For this review, take the finished solid that the model builds, in its own axes (mm). A direction names the side the tool comes from. Round coordinates to 2 decimals unless told otherwise and drop trailing zeros. Order: outer loops, then holes, each group sorted by start corner. A loop starts at its lowest first (then second) coordinate and runs counter-clockwise, first axis right, second up. Notation, with made-up numbers: (19.25, 82) -> (53.25, 82) arc R22 cw to (53.25, 113) -> close; hole circle Ø3 at (71, 87). An arc over 180 degrees is marked (long way). Use a Markdown table: item, result. Add a question column.
1) Machinability: for faces 5 (the face through (-34.3, -493, -43)), 6 (the face through (0, -493, -55)), 7 (the face through (3, -1000, -54)), which of the approach directions +Z, -Z, +X, -X, +Y, -Y give a long, thin tool a straight path to every point of the face, cutting with its end or side? Answer none if there is none.
2) Wall thickness on line 1 along X through (y, z) = (-635, -70); line 2 along X through (y, z) = (-332.5, -45); line 3 along X through (y, z) = (-213, -13.5): over which ranges is each line inside the solid? List them lowest first. Write a range as [from, to].
3) Clearance check with flat-ended pins moving along their axes: P1, Ø2.5, axis at x = -33, y = -698.5, coming from the -Z side; P2, Ø1.6, axis at x = -35, y = -397, coming from the +Z side; P3, Ø2, axis at y = -471.5, z = -89.5, coming from the +X side. State where each tip first meets the part, or that it passes through.
4) Draft analysis for pull direction Z (two halves, no side actions). For faces 1 (the face through (-27.1, -493, -80)), 2 (the face through (-7, -493, -28)), 3 (the face through (-17, -493, -92)), 4 (the face through (21, -493, -53)), state which applies: pulls with the +Z half, pulls with the -Z half, needs draft (parallel to the pull), parting line crosses it, or undercut.
5) Consider section A-A (z = -44). State the section outline as (x, y) points, plus the area to 3 significant figures.
```python
from build123d import *

# Parameters (mm, degrees)
F1_DEPTH = 1000
F2_R     = 0.5
F5_DEPTH = 1000


with BuildPart() as f1:
    # F0 (on Front) → F1 (new body)
    with BuildSketch(Plane.XZ):
        Polygon((0, -5), (0, -3), (-7, -3), (-7, -53), (-34.3, -53), (-34.3, -33), (-36.3, -33), (-36.3, -61.5), (-34.3, -61.5), (-34.3, -55), (-29.1, -55), (-29.1, -75), (-34.3, -75), (-34.3, -68.5), (-36.3, -68.5), (-36.3, -77), (-29.1, -77), (-29.1, -92), (-5, -92), (-5, -88), (-7, -88), (-7, -90), (-27.1, -90), (-27.1, -69.9), (-25.1, -69.9), (-25.1, -67.9), (-27.1, -67.9), (-27.1, -55), (0, -55), (0, -53), (-5, -53), (-5, -5), align=None)
    extrude(amount=F1_DEPTH)

    # F2
    f2_edges = [f1.edges().sort_by_distance(p)[0] for p in [
        (-36.3, -500, -33),
        (-36.3, -500, -68.5),
        (-5, -500, -92),
        (-5, -500, -88),
        (-7, -500, -3),
        (-34.3, -500, -33),
        (-5, -500, -53),
        (-25.1, -500, -67.9),
        (-29.1, -500, -92),
        (-36.3, -500, -77),
        (-36.3, -500, -61.5),
        (-7, -500, -53),
    ]]
    fillet(f2_edges, radius=F2_R)

    # F3: F1 across plane


with BuildPart() as f1_1:
    add(f1.part)
    add(f1.part.mirror(Plane.YZ))

    # F4 (on face) → F5 (cut)
    with BuildSketch(Plane.XZ.offset(1000)):
        Polygon((0, -3.5), (0, -3), (-0.83214, -3), align=None)
        Polygon((0.83214, -3), (0, -3), (0, -3.5), align=None)
    extrude(amount=-F5_DEPTH, mode=Mode.SUBTRACT)


solid = f1_1.part
```
Results list:
| question | item | result |
|---|---|---|
| 1 | face 5 | +Z, +Y, -Y |
| 1 | face 6 | +Y, -Y |
| 1 | face 7 | +Z, -Z, +X, -X, -Y |
| 2 | line 1 | [-36.3, -34.3], [-29.1, -27.1], [27.1, 29.1], [34.3, 36.3] |
| 2 | line 2 | [-36.3, -34.3], [-7, -5], [5, 7], [34.3, 36.3] |
| 2 | line 3 | [-7, -5], [5, 7] |
| 3 | P1 | z = -77 |
| 3 | P2 | z = -33 |
| 3 | P3 | x = 29.1 |
| 4 | face 1 | undercut |
| 4 | face 2 | needs draft |
| 4 | face 3 | pulls with the -Z half |
| 4 | face 4 | pulls with the +Z half |
| 5 | outline | (-36.3, -1000) -> (-34.3, -1000) -> (-34.3, 0) -> (-36.3, 0) -> close; (-7, -1000) -> (-5, -1000) -> (-5, 0) -> (-7, 0) -> close; (5, -1000) -> (7, -1000) -> (7, 0) -> (5, 0) -> close; (34.3, -1000) -> (36.3, -1000) -> (36.3, 0) -> (34.3, 0) -> close |
| 5 | area | 8,000 mm2 |
